Autodesk Inventor part; units mm, degrees
ref_plane "YZ Plane" through (0, 0, 0) normal (1, 0, 0) x (0, 1, 0)
ref_plane "XZ Plane" through (0, 0, 0) normal (0, 1, 0) x (-1, 0, 0)
ref_plane "XY Plane" through (0, 0, 0) normal (0, 0, 1) x (1, 0, 0)
sketch "Sketch1" plane through (0, 0, 0) normal (1, 0, 0) x (0, 1, 0)
  line L0 (0, 0) -> (0, -10) construction
  line L1 (0, -10) -> (0, -50) construction
  circle A0 centre (0, -10) radius 2
  circle A1 centre (0, -50) radius 2
  line L2 (10, 0) -> (10, -59)
  line L3 (10, -59) -> (0, -59)
  line L4 (0, -59) -> (-10, -59)
  line L5 (-10, -59) -> (-10, 0)
  line L6 (0, 0) -> (10, 0)
  line L7 (0, 0) -> (-10, 0)
  line L8 (0, -50) -> (0, -59) construction
  circle A2 centre (0, 40) radius 25
  line L9 (10, 0) -> (10, 10)
  line L10 (10, 10) -> (-10, 10)
  line L11 (-10, 10) -> (-10, 0)
  arc A3 (22.804878, 29.756098) -> (10, -30) centre (155.833333, -30) ccw
  arc A4 (-10, -30) -> (-22.804878, 29.756098) centre (-155.833333, -30) ccw
  line L12 (0, -30) -> (21, -30) construction
  line L13 (0, -30) -> (-21, -30) construction
  circle A5 centre (21, -30) radius 3.5
  circle A6 centre (-21, -30) radius 3.5
  circle A7 centre (21, -30) radius 10
  circle A8 centre (-21, -30) radius 10
  circle A9 centre (21, -30) radius 6.5
  circle A10 centre (-21, -30) radius 6.5
  line L14 (-10, -59) -> (-25, -59)
  line L15 (10, -59) -> (25, -59)
  arc A11 (-28.958574, -23.94516) -> (-22.804878, 29.756098) centre (-71.055556, 8.081996) ccw
  arc A12 (22.804878, 29.756098) -> (28.958574, -23.94516) centre (71.055556, 8.081996) ccw
  line L16 (0, 0) -> (15, 0)
  line L17 (10, 0) -> (25, 0)
  line L18 (25, -59) -> (25, -50.3)
  arc A13 (29.39318, -35.436408) -> (25, -50.3) centre (52.340833, -50.3) ccw
  line L19 (25, 0) -> (25, -8.7)
  arc A14 (25, -8.7) -> (29.529682, -24.780371) centre (55.8075, -8.7) ccw
  line L20 (-10, 0) -> (-25, 0)
  line L21 (-25, -59) -> (-25, -50.3)
  arc A15 (-25, -50.3) -> (-29.39318, -35.436408) centre (-52.340833, -50.3) ccw
  line L22 (-25, 0) -> (-25, -8.7)
  arc A16 (-29.529682, -24.780371) -> (-25, -8.7) centre (-55.8075, -8.7) ccw
  circle A17 centre (0, -50) radius 4
  circle A18 centre (0, -10) radius 4
  circle A19 centre (0, 40) radius 7.235
  circle A20 centre (0, 40) radius 5.08
  point P0 (-10, -30)
  point P1 (10, -30)
  point P2 (23.824594, -39.592793)
  point P3 (10, -63.33599)
  point P4 (-30.230769, -33.846154)
  point P5 (28.958574, -23.94516)
  point P6 (22.804878, 29.756098)
  point P7 (30.230769, -26.153846)
  point P8 (18.78151, 0)
  point P9 (-18.78151, 0)
  point P10 (-13.119069, 0)
  point P11 (-29.39318, -35.436408)
  dimension "d0" = 4
  dimension "d1" = 4
  dimension "d2" = 40
  dimension "d3" = 10
  dimension "d5" = 9
  dimension "d7" = 10
  dimension "d8" = 10
  dimension "d9" = 50
  dimension "d12" = 30
  dimension "d13" = 10
  dimension "d14" = 20
  dimension "d30" = 21
  dimension "d31" = 7
  dimension "d32" = 7
  dimension "d33" = 20
  dimension "d34" = 20
  dimension "d38" = 3
  dimension "d48" = 15
  dimension "d55" = 15
  dimension "d56" = 8.7
  dimension "d57" = 8.7
  dimension "d58" = 15
  dimension "d134" = 8
  dimension "d135" = 8
  dimension "d138" = 14.47
  dimension "d157" = 10.16
extrude "Extrusion1" add sketch "Sketch1" along normal blind 5 contours L16 A3 L2 | L2 L3 L4 L5 L7 L6 | L6 L7 L11 L10 L9 | L9 L10 L11 L20 A4 A2 A3 L16 | A3 L16 L17 A12 A7 A13 L18 L15 L2 | A3 A12 L17 L16 | L5 A4 L20 | A2 | L5 L14 L21 A15 A8 A11 L20 A4 | L20 A11 A4 | L17 L19 A14 A7 A12 | A11 A8 A16 L22 L20 | A7 | A8 | A5 | A6 | A9 | A10 | A17 | A18 | A19 | A20
fillet "Face Fillet1" radius 5 1 edges at (2.5, -18.7815, 0)
fillet "Face Fillet2" radius 5 1 edges at (2.5, 18.7815, 0)
extrude "Extrusion16" cut sketch "Sketch1" along normal up to surface (5 mm away) contours A20
extrude "Extrusion17" cut sketch "Sketch1" along normal blind 2 from surface at 0 contours A19 | A20
extrude "Extrusion11" cut sketch "Sketch1" against normal blind 2.5 from surface at 5 contours A17 | A18
extrude "Extrusion19" add sketch "Sketch1" against normal blind 15 contours A5 | A6
extrude "Extrusion20" add sketch "Sketch1" against normal blind 5 contours A9 | A10
fillet "Fillet4" radius 2 2 edges at (-15, 17.5, -30) (-15, -24.5, -30)
chamfer "Chamfer2" distance 2 angle 45 17 edges at (5, 0, 65) (5, -19.0046, 17.4944) (5, -19.8398, 1.3525) (5, -24.1298, 0) (5, 19.0046, 17.4944) (5, 19.8398, 1.3525) (5, 24.1298, 0) (5, 25, -4.35) (5, 26.154, -17.0531) (5, 30.9992, -30.1281) (5, 26.1213, -42.5504) (5, 25, -54.65) (5, -26.154, -17.0531) (5, -30.9992, -30.1281) (5, -26.1213, -42.5504) (5, -25, -54.65) (5, -25, -4.35)
sketch "Sketch15" plane through (0, 0, 0) normal (-1, 0, 0) x (0, 0, 1)
  line L0 (0, 25) -> (0, 23.259692)
  line L1 (0, 25) -> (-8, 25)
  line L2 (-8, 25) -> (-8, 22.5)
  line L3 (-8, 22.5) -> (0, 22.5)
  line L4 (0, 22.5) -> (0, 25)
  point P0 (0, 0)
  dimension "d175" = 8
  dimension "d176" = 2.5
extrude "Extrusion21" add sketch "Sketch15" along normal blind 8
sketch "Sketch16" plane through (0, 25, -8.7) normal (0, 1, 0) x (1, 0, 0)
  circle A0 centre (-4, -4.7) radius 2
  line L0 (-8, -8.7) -> (-8, -0.7)
  line L1 (-8, -8.7) -> (3, -8.7)
  point P0 (0, -8.7)
  dimension "d179" = 4
  dimension "d180" = 4
  dimension "d181" = 4
extrude "Extrusion22" cut sketch "Sketch16" against normal up to surface (2.5 mm away)
mirror "Mirror2" about plane through (0, 0, 0) normal (0, 1, 0) of "Extrusion22", "Extrusion21"
equation "\"d0\" = M4_HOLE_D"
equation "\"d1\" = d0"
equation "\"d14\" = 0.5 * d2"
equation "\"d32\" = d31"
equation "\"d34\" = d33"
equation "\"M4_HOLE_D\" = 4"
equation "\"M3_HOLE_D\" = 3"
equation "\"d88\" = 3"
properties part number "bearing_arm_3DPrint"
The listing builds one solid part. Answer for the finished solid, in the listing's coordinates (mm). A direction names the side the tool comes from. Round coordinates to 2 decimals unless told otherwise and drop trailing zeros. Write each loop counter-clockwise with the first axis right and the second up, starting at its lowest first coordinate (ties: lowest second). Pieces come first, ordered by that corner, then holes. Notation, with made-up numbers: (58, 14.5) - (83, 14.5) arc R32 ccw to (83, 44.5) - close; hole circle Ø10 at (-39.75, 24.5). An arc over 180 degrees is marked (long way). Use a Markdown table: item, result. Add a question column.
1. The part is cut by section A-A (z = 40). Write down the section's boundary in (x, y) (3 decimals).
2. A tool of negligible diameter and unlimited length cuts with its end or side. For faces 4 (the face through (-8.94, -21.46, -26.53)), 5 (the face through (-8, -24, -4)), 6 (the face through (3.768, -0.867, -13.905)), 7 (the face through (-2, -22.5, -3)), from which of +Z, -Z, +X, -X, +Y, -Y can it reach the whole face along a straight path? Write none if from no direction.
3. Consider line 1 (Z direction, x = 1.6, y = 0) (3 decimals); line 2 (Z direction, x = 4.45, y = 0); line 3 (X direction, y = 15, z = -50). Determine where each line is inside the solid, lowest interval first.
4. Flat-ended cylindrical pins translate along their axes: P1, Ø4.5, axis at x = -3, z = -3, coming from the +Y side; P2, Ø5, axis at x = -11.5, y = -16, coming from the -Z side; P3, Ø4.5, axis at y = 0, z = -50, coming from the -X side; P4, Ø23, axis at y = 0, z = 40, coming from the +X side. Find the tip coordinate at first contact, or state that the pin passes through.
5. The part is cut by section B-B (z = -4). Write down the section's boundary in (x, y), and give its area (3 significant figures).
6. The part is cut by section C-C (x = -10). Write down the section's boundary in (y, z), and give its area (3 significant figures).
7. For a pull along Z with two mould halves and no side action, classify faces 1 (the face through (1, -31, -30)), 2 (the face through (-15, -21, -30)), 3 (the face through (-4, 24, -8)) as +Z half, -Z half, draft (parallel to the pull), parting line (faces both ways), or undercut.
Reported:
| question | item | result |
|---|---|---|
| 1 | outline | (0, -25) - (3, -25) - (5, -23) - (5, -5.08) - (2, -5.08) - (2, -7.235) - (0, -7.235) - close; (0, 7.235) - (2, 7.235) - (2, 5.08) - (5, 5.08) - (5, 23) - (3, 25) - (0, 25) - close |
| 2 | face 4 | -X |
| 2 | face 5 | +Z, -X, +Y, -Y |
| 2 | face 6 | +X |
| 2 | face 7 | +Z, -X |
| 3 | line 1 | -59 to -52, -48 to -12, -8 to 32.765, 47.235 to 65 |
| 3 | line 2 | -59 to -54, -46 to -14, -6 to 34.92, 45.08 to 63.55 |
| 3 | line 3 | 0 to 5 |
| 4 | P1 | y = 25 |
| 4 | P2 | z = -32.45 |
| 4 | P3 | x = 0 |
| 4 | P4 | x = 5 |
| 5 | outline | (-8, -25) - (-6, -25) - (-6, -22.5) - (-8, -22.5) - close; (-8, 22.5) - (-6, 22.5) - (-6, 25) - (-8, 25) - close; (-2, -25) - (3, -25) - (5, -23) - (5, 23) - (3, 25) - (-2, 25) - (-2, 22.5) - (0, 22.5) - (0, -22.5) - (-2, -22.5) - close |
| 5 | area | 266 mm^2 |
| 6 | outline | circle Ø7 at (-21, -30); circle Ø7 at (21, -30) |
| 6 | area | 77.0 mm^2 |
| 7 | face 1 | parting line |
| 7 | face 2 | draft |
| 7 | face 3 | undercut |
